from build123d import *

# Parameters (mm, degrees)
ESBO_O1_W                = 66.94
ESBO_O1_H                = 40
RESSALTO_EXTRUS_O1_DEPTH = 9.5
ESBO_O2_W                = 7
ESBO_O2_H                = 40
RESSALTO_EXTRUS_O2_DEPTH = 50
ESBO_O3_W                = 28.44
ESBO_O3_H                = 40
RESSALTO_EXTRUS_O3_DEPTH = 8
RESSALTO_EXTRUS_O4_DEPTH = 2
RESSALTO_EXTRUS_O5_DEPTH = 6
FILETE1_R                = 5
FILETE2_R                = 20
ESBO_O6_R                = 1.65
CORTE_EXTRUS_O1_DEPTH    = 63.217786628
CORTE_EXTRUS_O2_DEPTH    = 8
FILETE4_R                = 6
CORTE_EXTRUS_O3_DEPTH    = 94.912194911


with BuildPart() as part:
    # Esboço1 → Ressalto-extrusão1 (new body)
    with BuildSketch(Plane.XY):
        with Locations((2.706874237, 0.253968254)):
            Rectangle(ESBO_O1_W, ESBO_O1_H)
    extrude(amount=RESSALTO_EXTRUS_O1_DEPTH)

    # Esboço2 → Ressalto-extrusão2 (add)
    with BuildSketch(Plane.XY.offset(9.5)):
        with Locations((32.676874237, 0.253968254)):
            Rectangle(ESBO_O2_W, ESBO_O2_H)
    extrude(amount=RESSALTO_EXTRUS_O2_DEPTH)

    # Esboço3 → Ressalto-extrusão3 (add)
    with BuildSketch(Plane.XY.offset(9.5)):
        with Locations((-16.543125763, 0.253968254)):
            Rectangle(ESBO_O3_W, ESBO_O3_H)
    extrude(amount=RESSALTO_EXTRUS_O3_DEPTH)

    # Esboço4 → Ressalto-extrusão4 (add)
    with BuildSketch(Plane.XZ.offset(19.746031746)):
        Polygon((-2.323125763, 9.5), (-2.323125763, 17.5), (-30.763125763, 17.5), (-30.763125763, 0), (36.176874237, 0), (36.176874237, 59.5), (29.176874237, 59.5), (29.176874237, 9.5), align=None)
    ressalto_extrus_o4 = extrude(amount=RESSALTO_EXTRUS_O4_DEPTH)

    # Espelhar1: Ressalto-extrusão4 across plane
    add(ressalto_extrus_o4.mirror(Plane.ZX.offset(0.253968254)))

    # Esboço5 → Ressalto-extrusão5 (add)
    with BuildSketch(Plane.XZ.offset(21.746031746)):
        with BuildLine():
            Line((36.176874237, 59.5), (29.176874237, 59.5))
            add(Edge.make_bspline(
                [(29.176874237, 59.5), (16.163128622, 21.143295095), (-30.763125763, 17.5)],
                knots=[0, 0, 0, 1, 1, 1], degree=2))
            Line((-30.763125763, 17.5), (-30.763125763, 0))
            Line((-30.763125763, 0), (36.176874237, 0))
            Line((36.176874237, 0), (36.176874237, 59.5))
        make_face()
    ressalto_extrus_o5 = extrude(amount=RESSALTO_EXTRUS_O5_DEPTH)

    # Espelhar2: Ressalto-extrusão5 across plane
    add(ressalto_extrus_o5.mirror(Plane.ZX.offset(0.253968254)))

    # Filete1
    filete1_edges = [part.edges().sort_by_distance(p)[0] for p in [
        (-2.323125763, 0.253968254, 17.5),
    ]]
    fillet(filete1_edges, radius=FILETE1_R)

    # Filete2
    filete2_edges = [part.edges().sort_by_distance(p)[0] for p in [
        (29.176874237, 0.253968254, 9.5),
    ]]
    fillet(filete2_edges, radius=FILETE2_R)

    # Esboço6 → Corte-extrusão1 (cut, through all)
    with BuildSketch(Plane.XY.offset(17.5)):
        with Locations((-19.323125763, 11.753968254)):
            Circle(ESBO_O6_R)
        with Locations((-19.323125763, 0.253968254)):
            Circle(ESBO_O6_R)
        with Locations((-19.323125763, -11.246031746)):
            Circle(ESBO_O6_R)
    extrude(amount=-CORTE_EXTRUS_O1_DEPTH, mode=Mode.SUBTRACT)

    # Esboço7 → Corte-extrusão2 (cut)
    with BuildSketch(Plane(origin=(0, 0, 0), x_dir=(-1, 0, 0), z_dir=(0, 0, -1))):
        with BuildLine():
            Line((27.323125763, 11.753968254), (27.323125763, -11.246031746))
            ThreePointArc((27.323125763, -11.246031746), (19.323125763, -19.246031746), (11.323125763, -11.246031746))
            Line((11.323125763, -11.246031746), (11.323125763, 11.753968254))
            ThreePointArc((11.323125763, 11.753968254), (19.323125763, 19.753968254), (27.323125763, 11.753968254))
        make_face()
    extrude(amount=-CORTE_EXTRUS_O2_DEPTH, mode=Mode.SUBTRACT)

    # Filete4
    filete4_edges = [part.edges().sort_by_distance(p)[0] for p in [
        (36.176874237, 28.253968254, 29.75),
        (-30.763125763, 28.253968254, 8.75),
        (-30.763125763, -27.746031746, 8.75),
        (36.176874237, -27.746031746, 29.75),
    ]]
    fillet(filete4_edges, radius=FILETE4_R)

    # Esboço8 → Corte-extrusão3 (cut, through all)
    with BuildSketch(Plane(origin=(36.176874237, 0, 0), x_dir=(0, 0, -1), z_dir=(1, 0, 0))):
        with BuildLine():
            Line((-53.6, 1.803968254), (-49.4, 1.803968254))
            ThreePointArc((-49.4, 1.803968254), (-47.85, 0.253968254), (-49.4, -1.296031746))
            Line((-49.4, -1.296031746), (-53.6, -1.296031746))
            ThreePointArc((-53.6, -1.296031746), (-55.15, 0.253968254), (-53.6, 1.803968254))
        make_face()
        with BuildLine():
            Line((-40.55, -14.346031746), (-40.55, -10.146031746))
            ThreePointArc((-40.55, -10.146031746), (-39, -8.596031746), (-37.45, -10.146031746))
            Line((-37.45, -10.146031746), (-37.45, -14.346031746))
            ThreePointArc((-37.45, -14.346031746), (-39, -15.896031746), (-40.55, -14.346031746))
        make_face()
        with BuildLine():
            Line((-24.4, -1.296031746), (-28.6, -1.296031746))
            ThreePointArc((-28.6, -1.296031746), (-30.15, 0.253968254), (-28.6, 1.803968254))
            Line((-28.6, 1.803968254), (-24.4, 1.803968254))
            ThreePointArc((-24.4, 1.803968254), (-22.85, 0.253968254), (-24.4, -1.296031746))
        make_face()
        with BuildLine():
            Line((-37.45, 14.853968254), (-37.45, 10.653968254))
            ThreePointArc((-37.45, 10.653968254), (-39, 9.103968254), (-40.55, 10.653968254))
            Line((-40.55, 10.653968254), (-40.55, 14.853968254))
            ThreePointArc((-40.55, 14.853968254), (-39, 16.403968254), (-37.45, 14.853968254))
        make_face()
    extrude(amount=-CORTE_EXTRUS_O3_DEPTH, mode=Mode.SUBTRACT)


solid = part.part
For this review, take the finished solid that the model builds, in its own axes (mm). A direction names the side the tool comes from. Coordinates: 2 decimals unless noted, no trailing zeros. Order: outer loops, then holes, each group sorted by start corner. A loop starts at its lowest first (then second) coordinate and runs counter-clockwise, first axis right, second up. Notation, with made-up numbers: (17.25, 37) -> (75.25, 37) arc R26 cw to (75.25, 59) -> close; hole circle Ø1 at (-26.5, -3). An arc over 180 degrees is marked (long way). Return JSON: item names as keys, results as strings.
1. For line 1 (Y direction, x = 28, z = 41); line 2 (Z direction, x = 32, y = 15); line 3 (X direction, y = 5.5, z = 5), list the stretches that pass through material, from the lowest coordinate up. Write a range as from..to.
Answer block:
{"line 1": "-27.75..-21.75, 22.25..28.25", "line 2": "0..37.46, 40.54..59.5", "line 3": "-30.76..-27.32, -11.32..36.18"}
2. For pin 1 Ø9 at (y, z) = (-7.5, 38.5) entering from -X; pin 2 Ø2 at (x, z) = (33.5, 51) entering from -Y; pin 3 Ø2 at (x, y) = (17.5, 22) entering from +Z; pin 4 Ø1 at (x, y) = (1, 0) entering from -Z, all flat-tipped, find the tip position at first contact; note any pin that passes through.
Answer block:
{"pin 1": "x = 29.18", "pin 2": "y = -27.28", "pin 3": "z = 39.79", "pin 4": "z = 0"}
3. We need section A-A on y = 3. Write out the cut boundary in (x, z).
Answer block:
{"outline": "(-30.76, 0) -> (-27.32, 0) -> (-27.32, 8) -> (-11.32, 8) -> (-11.32, 0) -> (36.18, 0) -> (36.18, 59.5) -> (29.18, 59.5) -> (29.18, 29.5) arc R20 cw to (9.18, 9.5) -> (-2.32, 9.5) -> (-2.32, 12.5) arc R5 ccw to (-7.32, 17.5) -> (-30.76, 17.5) -> close"}
4. The part is to be moulded in two halves that separate along Z. For faces 1 (the cylindrical face through (32.726, 16.404, 39.034)), 2 (the flat face through (-21, 1, 8)), 3 (the flat face through (-11.323, 0, 4)), say which applies: +Z half, -Z half, draft (parallel to the pull), parting line (faces both ways), or undercut.
Answer block:
{"face 1": "undercut", "face 2": "-Z half", "face 3": "draft"}
5. Machinability: for faces 4 (the cylindrical face through (-3.827, -0.054, 16.074)), 5 (the flat face through (33, 13, 37.45)), 6 (the cylindrical face through (-20.97, 0.33, 12.82)), 7 (the flat face through (29.177, 0, 45)), 8 (the cylindrical face through (-19.147, 19.752, 3.944)), which of the approach directions +Z, -Z, +X, -X, +Y, -Y give a long, thin tool a straight path to every point of the face, cutting with its end or side? Answer none if there is none.
Answer block:
{"face 4": "+Z", "face 5": "+X, -X", "face 6": "+Z, -Z", "face 7": "+Z, -X", "face 8": "-Z"}
6. We need section B-B on x = -20. State how many separate pieces and enclosed holes the cut face has, and give its area (3 significant figures).
Answer block:
{"separate pieces": "4", "enclosed holes": "0", "area": "599 mm²"}
